```python
from build123d import *

# Parameters (mm, degrees)
BOSS_EXTRUDE1_DEPTH = 10
BOSS_EXTRUDE2_DEPTH = 10
SKETCH3_W           = 40
SKETCH3_H           = 10
BOSS_EXTRUDE3_DEPTH = 10


with BuildPart() as part:
    # Sketch1 → Boss-Extrude1 (new body)
    with BuildSketch(Plane.XY):
        with BuildLine():
            ThreePointArc((0.378650208, 9.55600532), (0, 9.736842105), (-0.378650208, 9.55600532))
            ThreePointArc((-0.378650208, 9.55600532), (-0.641665483, 9.327218092), (-0.967233833, 9.202615203))
            ThreePointArc((-0.967233833, 9.202615203), (-1.311594131, 9.256805753), (-1.616429431, 9.425909481))
            ThreePointArc((-1.616429431, 9.425909481), (-2.024403305, 9.524068744), (-2.357181016, 9.268457871))
            ThreePointArc((-2.357181016, 9.268457871), (-2.566881237, 8.989986242), (-2.85942874, 8.800416759))
            ThreePointArc((-2.85942874, 8.800416759), (-3.207530788, 8.781826585), (-3.540863348, 8.883856167))
            ThreePointArc((-3.540863348, 8.883856167), (-3.960330472, 8.895047877), (-4.232691702, 8.575834338))
            ThreePointArc((-4.232691702, 8.575834338), (-4.379911963, 8.259848855), (-4.62665289, 8.013597874))
            ThreePointArc((-4.62665289, 8.013597874), (-4.963282959, 7.923039454), (-5.310544545, 7.95353571))
            ThreePointArc((-5.310544545, 7.95353571), (-5.723172193, 7.877270735), (-5.923213451, 7.508405694))
            ThreePointArc((-5.923213451, 7.508405694), (-6.00151952, 7.168716439), (-6.191670107, 6.876546309))
            ThreePointArc((-6.191670107, 6.876546309), (-6.502115847, 6.717977481), (-6.848129462, 6.675607576))
            ThreePointArc((-6.848129462, 6.675607576), (-7.235883827, 6.515219062), (-7.354862349, 6.112823691))
            ThreePointArc((-7.354862349, 6.112823691), (-7.360831875, 5.764276714), (-7.48608163, 5.438956672))
            ThreePointArc((-7.48608163, 5.438956672), (-7.756775072, 5.219307655), (-8.086418262, 5.105923359))
            ThreePointArc((-8.086418262, 5.105923359), (-8.432352616, 4.868421053), (-8.465068469, 4.450081961))
            ThreePointArc((-8.465068469, 4.450081961), (-8.398440555, 4.107910437), (-8.453315463, 3.76365853))
            ThreePointArc((-8.453315463, 3.76365853), (-8.672426006, 3.492529039), (-8.97129178, 3.31308579))
            ThreePointArc((-8.97129178, 3.31308579), (-9.260287132, 3.008849682), (-9.205310478, 2.592850295))
            ThreePointArc((-9.205310478, 2.592850295), (-9.068997084, 2.272008762), (-9.051098847, 1.92387045))
            ThreePointArc((-9.051098847, 1.92387045), (-9.209050308, 1.613110146), (-9.464076798, 1.375450473))
            ThreePointArc((-9.464076798, 1.375450473), (-9.683502665, 1.017777142), (-9.543236247, 0.622298629))
            ThreePointArc((-9.543236247, 0.622298629), (-9.343194922, 0.336809401), (-9.25330578, 0))
            ThreePointArc((-9.25330578, 0), (-9.343194922, -0.336809401), (-9.543236247, -0.622298629))
            ThreePointArc((-9.543236247, -0.622298629), (-9.683502665, -1.017777142), (-9.464076798, -1.375450473))
            ThreePointArc((-9.464076798, -1.375450473), (-9.209050308, -1.613110146), (-9.051098847, -1.92387045))
            ThreePointArc((-9.051098847, -1.92387045), (-9.068997084, -2.272008762), (-9.205310478, -2.592850295))
            ThreePointArc((-9.205310478, -2.592850295), (-9.260287132, -3.008849682), (-8.97129178, -3.31308579))
            ThreePointArc((-8.97129178, -3.31308579), (-8.672426006, -3.492529039), (-8.453315463, -3.76365853))
            ThreePointArc((-8.453315463, -3.76365853), (-8.398440555, -4.107910437), (-8.465068469, -4.450081961))
            ThreePointArc((-8.465068469, -4.450081961), (-8.432352616, -4.868421053), (-8.086418262, -5.105923359))
            ThreePointArc((-8.086418262, -5.105923359), (-7.756775072, -5.219307655), (-7.48608163, -5.438956672))
            ThreePointArc((-7.48608163, -5.438956672), (-7.360831875, -5.764276714), (-7.354862349, -6.112823691))
            ThreePointArc((-7.354862349, -6.112823691), (-7.235883827, -6.515219062), (-6.848129462, -6.675607576))
            ThreePointArc((-6.848129462, -6.675607576), (-6.502115847, -6.717977481), (-6.191670107, -6.876546309))
            ThreePointArc((-6.191670107, -6.876546309), (-6.00151952, -7.168716439), (-5.923213451, -7.508405694))
            ThreePointArc((-5.923213451, -7.508405694), (-5.723172193, -7.877270735), (-5.310544545, -7.95353571))
            ThreePointArc((-5.310544545, -7.95353571), (-4.963282959, -7.923039454), (-4.62665289, -8.013597874))
            ThreePointArc((-4.62665289, -8.013597874), (-4.379911963, -8.259848855), (-4.232691702, -8.575834338))
            ThreePointArc((-4.232691702, -8.575834338), (-3.960330472, -8.895047877), (-3.540863348, -8.883856167))
            ThreePointArc((-3.540863348, -8.883856167), (-3.207530788, -8.781826585), (-2.85942874, -8.800416759))
            ThreePointArc((-2.85942874, -8.800416759), (-2.566881237, -8.989986242), (-2.357181016, -9.268457871))
            ThreePointArc((-2.357181016, -9.268457871), (-2.024403305, -9.524068744), (-1.616429431, -9.425909481))
            ThreePointArc((-1.616429431, -9.425909481), (-1.311594131, -9.256805753), (-0.967233833, -9.202615203))
            ThreePointArc((-0.967233833, -9.202615203), (-0.641665483, -9.327218092), (-0.378650208, -9.55600532))
            ThreePointArc((-0.378650208, -9.55600532), (0, -9.736842105), (0.378650208, -9.55600532))
            ThreePointArc((0.378650208, -9.55600532), (0.641665483, -9.327218092), (0.967233833, -9.202615203))
            ThreePointArc((0.967233833, -9.202615203), (1.311594131, -9.256805753), (1.616429431, -9.425909481))
            ThreePointArc((1.616429431, -9.425909481), (2.024403305, -9.524068744), (2.357181016, -9.268457871))
            ThreePointArc((2.357181016, -9.268457871), (2.566881237, -8.989986242), (2.85942874, -8.800416759))
            ThreePointArc((2.85942874, -8.800416759), (3.207530788, -8.781826585), (3.540863348, -8.883856167))
            ThreePointArc((3.540863348, -8.883856167), (3.960330472, -8.895047877), (4.232691702, -8.575834338))
            ThreePointArc((4.232691702, -8.575834338), (4.379911963, -8.259848855), (4.62665289, -8.013597874))
            ThreePointArc((4.62665289, -8.013597874), (4.963282959, -7.923039454), (5.310544545, -7.95353571))
            ThreePointArc((5.310544545, -7.95353571), (5.723172193, -7.877270735), (5.923213451, -7.508405694))
            ThreePointArc((5.923213451, -7.508405694), (6.00151952, -7.168716439), (6.191670107, -6.876546309))
            ThreePointArc((6.191670107, -6.876546309), (6.502115847, -6.717977481), (6.848129462, -6.675607576))
            ThreePointArc((6.848129462, -6.675607576), (7.235883827, -6.515219062), (7.354862349, -6.112823691))
            ThreePointArc((7.354862349, -6.112823691), (7.360831875, -5.764276714), (7.48608163, -5.438956672))
            ThreePointArc((7.48608163, -5.438956672), (7.756775072, -5.219307655), (8.086418262, -5.105923359))
            ThreePointArc((8.086418262, -5.105923359), (8.432352616, -4.868421053), (8.465068469, -4.450081961))
            ThreePointArc((8.465068469, -4.450081961), (8.398440555, -4.107910437), (8.453315463, -3.76365853))
            ThreePointArc((8.453315463, -3.76365853), (8.672426006, -3.492529039), (8.97129178, -3.31308579))
            ThreePointArc((8.97129178, -3.31308579), (9.260287132, -3.008849682), (9.205310478, -2.592850295))
            ThreePointArc((9.205310478, -2.592850295), (9.068997084, -2.272008762), (9.051098847, -1.92387045))
            ThreePointArc((9.051098847, -1.92387045), (9.209050308, -1.613110146), (9.464076798, -1.375450473))
            ThreePointArc((9.464076798, -1.375450473), (9.683502665, -1.017777142), (9.543236247, -0.622298629))
            ThreePointArc((9.543236247, -0.622298629), (9.343194922, -0.336809401), (9.25330578, 0))
            ThreePointArc((9.25330578, 0), (9.343194922, 0.336809401), (9.543236247, 0.622298629))
            ThreePointArc((9.543236247, 0.622298629), (9.683502665, 1.017777142), (9.464076798, 1.375450473))
            ThreePointArc((9.464076798, 1.375450473), (9.209050308, 1.613110146), (9.051098847, 1.92387045))
            ThreePointArc((9.051098847, 1.92387045), (9.068997084, 2.272008762), (9.205310478, 2.592850295))
            ThreePointArc((9.205310478, 2.592850295), (9.260287132, 3.008849682), (8.97129178, 3.31308579))
            ThreePointArc((8.97129178, 3.31308579), (8.672426006, 3.492529039), (8.453315463, 3.76365853))
            ThreePointArc((8.453315463, 3.76365853), (8.398440555, 4.107910437), (8.465068469, 4.450081961))
            ThreePointArc((8.465068469, 4.450081961), (8.432352616, 4.868421053), (8.086418262, 5.105923359))
            ThreePointArc((8.086418262, 5.105923359), (7.756775072, 5.219307655), (7.48608163, 5.438956672))
            ThreePointArc((7.48608163, 5.438956672), (7.360831875, 5.764276714), (7.354862349, 6.112823691))
            ThreePointArc((7.354862349, 6.112823691), (7.235883827, 6.515219062), (6.848129462, 6.675607576))
            ThreePointArc((6.848129462, 6.675607576), (6.502115847, 6.717977481), (6.191670107, 6.876546309))
            ThreePointArc((6.191670107, 6.876546309), (6.00151952, 7.168716439), (5.923213451, 7.508405694))
            ThreePointArc((5.923213451, 7.508405694), (5.723172193, 7.877270735), (5.310544545, 7.95353571))
            ThreePointArc((5.310544545, 7.95353571), (4.963282959, 7.923039454), (4.62665289, 8.013597874))
            ThreePointArc((4.62665289, 8.013597874), (4.379911963, 8.259848855), (4.232691702, 8.575834338))
            ThreePointArc((4.232691702, 8.575834338), (3.960330472, 8.895047877), (3.540863348, 8.883856167))
            ThreePointArc((3.540863348, 8.883856167), (3.207530788, 8.781826585), (2.85942874, 8.800416759))
            ThreePointArc((2.85942874, 8.800416759), (2.566881237, 8.989986242), (2.357181016, 9.268457871))
            ThreePointArc((2.357181016, 9.268457871), (2.024403305, 9.524068744), (1.616429431, 9.425909481))
            ThreePointArc((1.616429431, 9.425909481), (1.311594131, 9.256805753), (0.967233833, 9.202615203))
            ThreePointArc((0.967233833, 9.202615203), (0.641665483, 9.327218092), (0.378650208, 9.55600532))
        make_face()
    extrude(amount=BOSS_EXTRUDE1_DEPTH)

    # Sketch2 → Boss-Extrude2 (add)
    with BuildSketch(Plane(origin=(0, 0, 0), x_dir=(-1, 0, 0), z_dir=(0, 0, -1))):
        with BuildLine():
            Line((-20, 0), (-20, -30.991945279))
            Line((-20, -30.991945279), (20, -30.991945279))
            Line((20, -30.991945279), (20, 0))
            ThreePointArc((20, 0), (0, 20), (-20, 0))
        make_face()
    boss_extrude2 = extrude(amount=BOSS_EXTRUDE2_DEPTH)

    # Mirror2: Boss-Extrude2 across plane
    add(boss_extrude2.mirror(Plane.XY.offset(5)))

    # Sketch3 → Boss-Extrude3 (add)
    with BuildSketch(Plane(origin=(0, 0, 10), x_dir=(-1, 0, 0), z_dir=(0, 0, -1))):
        with Locations((0, -25.991945279)):
            Rectangle(SKETCH3_W, SKETCH3_H)
    extrude(amount=BOSS_EXTRUDE3_DEPTH)


solid = part.part
```
Check sheet for the modelled part. Datum: model origin and axes. Units: mm. A direction names the side the tool comes from. Coordinates: 2 decimals unless noted, no trailing zeros. Order: outer loops, then holes, each group sorted by start corner. A loop starts at its lowest first (then second) coordinate and runs counter-clockwise, first axis right, second up. Notation, with made-up numbers: M 49,-10.5 L 59,-10.5 A11 ccw 59,-5.5 Z; hole C 9,48.25 d2. An arc over 180 degrees is marked long. Write each question's results on one line, items separated by ' | '. Start each with the question number.
1. Material ranges on probe 1 along Z at (x, y) = (-15.5, -13); probe 2 along Y at (x, z) = (2, 4.5); probe 3 along Y at (x, z) = (9, 8.75), recorded low to high.
2. Cross-section at A-A on y = -13. Record the cut outline in (x, z).
3. Go/stop test with flat-tipped pins: P1, Ø2, axis at x = -15.5, z = 7, coming from the +Y side; P2, Ø12, axis at x = -4, z = 12.5, coming from the +Y side; P3, Ø8, axis at x = -1, z = 5.5, coming from the +Y side; P4, Ø6, axis at y = -16.5, z = 8, coming from the -X side. Record where each tip stops, or that it passes through.
4. Mould release check, pull along Y, two halves, no side actions. Record for faces 3 (the face through (0, -5, -10)), 4 (the face through (0, 20, -5)), 5 (the face through (0, -20.992, 5)), 6 (the face through (-4.2, -9.3, 10)): +Y half, -Y half, draft (parallel to the pull), parting line (faces both ways), or undercut.
5. Access from +Z, -Z, +X, -X, +Y, -Y to the whole of each face (thin tool, end or side, straight path). Record for faces 1 (the face through (0, -30.992, 5)), 2 (the face through (-4.2, -9.3, 0)).
6. Cross-section at B-B on x = 13. Record the cut outline in (y, z).
7. Cross-section at C-C on z = -2.75. Record the cut outline in (x, y), and give its area (3 significant figures).
Checks:
1) probe 1: z = -10 to 0, 10 to 20 | probe 2: y = -30.99 to -20.99, -9.53 to 9.53 | probe 3: y = -30.99 to -20.99, -3.3 to 3.3
2) outline: M -20,-10 L 20,-10 L 20,0 L -20,0 Z; M -20,10 L 20,10 L 20,20 L -20,20 Z
3) P1: stops at y = -20.99 | P2: stops at y = 20 | P3: stops at y = 9.74 | P4: stops at x = -20
4) face 3: draft | face 4: +Y half | face 5: undercut | face 6: undercut
5) face 1: +Z, -Z, +X, -X, -Y | face 2: none
6) outline: M -30.99,-10 L 15.2,-10 L 15.2,0 L -20.99,0 L -20.99,10 L 15.2,10 L 15.2,20 L -30.99,20 Z
7) outline: M -20,-30.99 L 20,-30.99 L 20,0 A20 ccw -20,0 Z | area: 1,870 mm²
